```python
from build123d import *

# Parameters (mm, degrees)
SKETCH1_W           = 32
SKETCH1_H           = 26
SKETCH1_R           = 2
BOSS_EXTRUDE1_DEPTH = 1
FILLET1_R           = 4
FILLET2_R           = 4
SKETCH2_W           = 32
SKETCH2_H           = 1
BOSS_EXTRUDE2_DEPTH = 25
FILLET3_R           = 4
FILLET4_R           = 4
SKETCH3_R           = 2
CUT_EXTRUDE1_DEPTH  = 40.458839314
FILLET5_R           = 0.5
FILLET6_R           = 0.5
FILLET7_R           = 0.5


with BuildPart() as part:
    # Sketch1 → Boss-Extrude1 (new body)
    with BuildSketch(Plane(origin=(0, 0, 0), x_dir=(1, 0, 0), z_dir=(0, 1, 0))):
        Rectangle(SKETCH1_W, SKETCH1_H)
        with Locations(Location((-8, -9, 0), (0, 0, 270))):
            Circle(SKETCH1_R, mode=Mode.SUBTRACT)
        with Locations(Location((7.905303365, -9, 0), (0, 0, 270))):
            Circle(SKETCH1_R, mode=Mode.SUBTRACT)
    extrude(amount=BOSS_EXTRUDE1_DEPTH)

    # Fillet1
    fillet1_edges = [part.edges().sort_by_distance(p)[0] for p in [
        (-16, 0.5, 13),
    ]]
    fillet(fillet1_edges, radius=FILLET1_R)

    # Fillet2
    fillet2_edges = [part.edges().sort_by_distance(p)[0] for p in [
        (16, 0.5, 13),
    ]]
    fillet(fillet2_edges, radius=FILLET2_R)

    # Sketch2 → Boss-Extrude2 (add)
    with BuildSketch(Plane(origin=(0, 1, 0), x_dir=(1, 0, 0), z_dir=(0, 1, 0))):
        with Locations((0, 12.5)):
            Rectangle(SKETCH2_W, SKETCH2_H)
    extrude(amount=BOSS_EXTRUDE2_DEPTH)

    # Fillet3
    fillet3_edges = [part.edges().sort_by_distance(p)[0] for p in [
        (16, 26, -12.5),
    ]]
    fillet(fillet3_edges, radius=FILLET3_R)

    # Fillet4
    fillet4_edges = [part.edges().sort_by_distance(p)[0] for p in [
        (-16, 26, -12.5),
    ]]
    fillet(fillet4_edges, radius=FILLET4_R)

    # Sketch3 → Cut-Extrude1 (cut, through all)
    with BuildSketch(Plane.XY.offset(-12)):
        with Locations((-8, 22)):
            Circle(SKETCH3_R)
        with Locations((8, 22)):
            Circle(SKETCH3_R)
    extrude(amount=-CUT_EXTRUDE1_DEPTH, mode=Mode.SUBTRACT)

    # Fillet5
    fillet5_edges = [part.edges().sort_by_distance(p)[0] for p in [
        (16, 11.5, -12),
        (14.828427125, 24.828427125, -12),
        (0, 26, -12),
        (-16, 11.5, -12),
        (-14.828427125, 24.828427125, -12),
    ]]
    fillet(fillet5_edges, radius=FILLET5_R)

    # Fillet6
    fillet6_edges = [part.edges().sort_by_distance(p)[0] for p in [
        (16, 1, -1.75),
        (14.828427125, 1, 11.828427125),
        (0, 1, 13),
        (-14.828427125, 1, 11.828427125),
        (-16, 1, -1.75),
    ]]
    fillet(fillet6_edges, radius=FILLET6_R)

    # Fillet7
    fillet7_edges = [part.edges().sort_by_distance(p)[0] for p in [
        (0, 0, -13),
    ]]
    fillet(fillet7_edges, radius=FILLET7_R)


solid = part.part
```
The model under review builds one solid part; all positions refer to its coordinate system, in mm. A direction names the side the tool comes from. Coordinates: 2 decimals unless noted, no trailing zeros. Order: outer loops, then holes, each group sorted by start corner. A loop starts at its lowest first (then second) coordinate and runs counter-clockwise, first axis right, second up. Notation, with made-up numbers: M 48.25,86 L 104.25,86 A20 cw 104.25,99 Z; hole C 31,53.5 d7. An arc over 180 degrees is marked long. One line per question, with ' | ' between items.
(1) Insertion check: pin 1 (3 mm diameter, centred on x = 1, y = 23, fed in from +Z); pin 2 (3.5 mm diameter, centred on x = 8, y = 22, fed in from -Z); pin 3 (4.5 mm diameter, centred on x = -8, z = 9, fed in from +Y). Each pin has a flat end and moves straight along its axis. Give the tip position at first contact, or say it passes through.
Geometry results:
pin 1: stops at z = -12 | pin 2: passes through | pin 3: stops at y = 1
(2) The part is to be moulded in two halves that separate along Y. For faces 3 (the face through (-9.6, 20.8, -12.5)), 4 (the face through (-14.859, 0.254, 11.797)), 5 (the face through (0, 0, 0)), 6 (the face through (0, 1, 0)), say which applies: +Y half, -Y half, draft (parallel to the pull), parting line (faces both ways), or undercut.
Geometry results:
face 3: undercut | face 4: draft | face 5: -Y half | face 6: +Y half
(3) Add section A-A, the plane x = -8. Write out the cut boundary in (y, z), then the cut area to 3 significant figures.
Geometry results:
outline: M 0,-12.5 A0.5 ccw 0.5,-13 L 20,-13 L 20,-12 L 1,-12 L 1,7 L 0,7 Z; M 0,11 L 1,11 L 1,12.5 A0.5 ccw 0.5,13 L 0,13 Z; M 24,-13 L 26,-13 L 26,-12.5 A0.5 ccw 25.5,-12 L 24,-12 Z | area: 42.8 mm²
(4) Add section B-B, the plane x = 0. Write out the cut boundary in (y, z), then the cut area to 3 significant figures.
Geometry results:
outline: M 0,-12.5 A0.5 ccw 0.5,-13 L 26,-13 L 26,-12.5 A0.5 ccw 25.5,-12 L 1,-12 L 1,12.5 A0.5 ccw 0.5,13 L 0,13 Z | area: 50.8 mm²
(5) Machinability: for faces 1 (the face through (0, 13, -12)), 2 (the face through (5.953, 0.493, 8.566)), which of the approach directions +Z, -Z, +X, -X, +Y, -Y give a long, thin tool a straight path to every point of the face, cutting with its end or side? Answer none if there is none.
Geometry results:
face 1: +Z, +X, -X, +Y | face 2: +Y, -Y
(6) For probe 1 along X at (y, z) = (0.45, 9); probe 2 along Y at (x, z) = (9.5, -8.75); probe 3 along Z at (x, y) = (12, 19.5), list the stretches that pass through material, from the lowest coordinate up. Write a range as from..to.
Geometry results:
probe 1: x = -16..-10, -6..5.91, 9.91..16 | probe 2: y = 0..1 | probe 3: z = -13..-12
(7) Add section D-D, the plane y = 4.75. Write out the cut boundary in (x, z), then the cut area to 3 significant figures.
Geometry results:
outline: M -16,-13 L 16,-13 L 16,-12.5 A0.5 ccw 15.5,-12 L -15.5,-12 A0.5 ccw -16,-12.5 Z | area: 31.9 mm²
(8) Add section C-C, the plane z = -7. Write out the cut boundary in (x, y).
Geometry results:
outline: M -16,0 L 16,0 L 16,0.5 A0.5 ccw 15.5,1 L -15.5,1 A0.5 ccw -16,0.5 Z
